```python
from build123d import *

# Parameters (mm, degrees)
SKIZZE2_W                       = 315
SKIZZE2_H                       = 50
AUFSATZ_LINEAR_AUSTRAGEN1_DEPTH = 85
SKIZZE4_W                       = 295
SKIZZE4_H                       = 55
SCHNITT_LINEAR_AUSTRAGEN1_DEPTH = 30
VERRUNDUNG1_R                   = 10
VERRUNDUNG2_R                   = 10
VERRUNDUNG3_R                   = 10
VERRUNDUNG4_R                   = 10
SKIZZE11_W                      = 45
SKIZZE11_H                      = 5
SKIZZE11_H_2                    = 5.008661904
SCHNITT_LINEAR_AUSTRAGEN4_DEPTH = 1.6
SKIZZE13_W                      = 295
SKIZZE13_H                      = 3
AUFSATZ_LINEAR_AUSTRAGEN2_DEPTH = 4.2
SKIZZE14_W                      = 8
SKIZZE14_H                      = 4
SCHNITT_LINEAR_AUSTRAGEN5_DEPTH = 19
SKIZZE15_W                      = 50
SKIZZE15_H                      = 1.5
AUFSATZ_LINEAR_AUSTRAGEN3_DEPTH = 2
SKIZZE16_W                      = 50
SKIZZE16_H                      = 1.5
AUFSATZ_LINEAR_AUSTRAGEN4_DEPTH = 2
SKIZZE17_R                      = 2.3
SCHNITT_LINEAR_AUSTRAGEN6_DEPTH = 4
SKIZZE19_W                      = 182.800022846
SKIZZE19_H                      = 85
SCHNITT_LINEAR_AUSTRAGEN8_DEPTH = 80


with BuildPart() as part:
    # Skizze2 → Aufsatz-Linear austragen1 (new body)
    with BuildSketch(Plane.XY):
        with Locations((157.5, 25)):
            Rectangle(SKIZZE2_W, SKIZZE2_H)
    extrude(amount=AUFSATZ_LINEAR_AUSTRAGEN1_DEPTH)

    # Skizze4 → Schnitt-Linear austragen1 (cut)
    with BuildSketch(Plane(origin=(0, 50, 0), x_dir=(1, 0, 0), z_dir=(0, 1, 0))):
        with Locations((157.5, -42.5)):
            Rectangle(SKIZZE4_W, SKIZZE4_H)
    extrude(amount=-SCHNITT_LINEAR_AUSTRAGEN1_DEPTH, mode=Mode.SUBTRACT)

    # Verrundung1
    verrundung1_edges = [part.edges().sort_by_distance(p)[0] for p in [
        (315, 25, 0),
    ]]
    fillet(verrundung1_edges, radius=VERRUNDUNG1_R)

    # Verrundung2
    verrundung2_edges = [part.edges().sort_by_distance(p)[0] for p in [
        (315, 25, 85),
    ]]
    fillet(verrundung2_edges, radius=VERRUNDUNG2_R)

    # Verrundung3
    verrundung3_edges = [part.edges().sort_by_distance(p)[0] for p in [
        (0, 25, 85),
    ]]
    fillet(verrundung3_edges, radius=VERRUNDUNG3_R)

    # Verrundung4
    verrundung4_edges = [part.edges().sort_by_distance(p)[0] for p in [
        (0, 25, 0),
    ]]
    fillet(verrundung4_edges, radius=VERRUNDUNG4_R)

    # Skizze11 → Schnitt-Linear austragen4 (cut)
    with BuildSketch(Plane(origin=(0, 50, 0), x_dir=(1, 0, 0), z_dir=(0, 1, 0))):
        with Locations((32.5, -12.5)):
            Rectangle(SKIZZE11_W, SKIZZE11_H)
        with Locations((32.5, -72.5)):
            Rectangle(SKIZZE11_W, SKIZZE11_H)
        with Locations((82.5, -72.5)):
            Rectangle(SKIZZE11_W, SKIZZE11_H)
        with Locations((132.5, -72.504330952)):
            Rectangle(SKIZZE11_W, SKIZZE11_H_2)
        with Locations((182.5, -72.504330952)):
            Rectangle(SKIZZE11_W, SKIZZE11_H_2)
        with Locations((232.5, -72.5)):
            Rectangle(SKIZZE11_W, SKIZZE11_H)
        with Locations((282.5, -72.5)):
            Rectangle(SKIZZE11_W, SKIZZE11_H)
        with Locations((282.5, -12.5)):
            Rectangle(SKIZZE11_W, SKIZZE11_H)
        with Locations((232.5, -12.5)):
            Rectangle(SKIZZE11_W, SKIZZE11_H)
        with Locations((182.5, -12.5)):
            Rectangle(SKIZZE11_W, SKIZZE11_H)
        with Locations((132.5, -12.5)):
            Rectangle(SKIZZE11_W, SKIZZE11_H)
        with Locations((82.5, -12.5)):
            Rectangle(SKIZZE11_W, SKIZZE11_H)
    extrude(amount=-SCHNITT_LINEAR_AUSTRAGEN4_DEPTH, mode=Mode.SUBTRACT)

    # Skizze13 → Aufsatz-Linear austragen2 (add)
    with BuildSketch(Plane(origin=(0, 20, 0), x_dir=(1, 0, 0), z_dir=(0, 1, 0))):
        with Locations((157.5, -68.5)):
            Rectangle(SKIZZE13_W, SKIZZE13_H)
    extrude(amount=AUFSATZ_LINEAR_AUSTRAGEN2_DEPTH)

    # Skizze14 → Schnitt-Linear austragen5 (cut)
    with BuildSketch(Plane.ZY.offset(-305)):
        with Locations((35, 24.4)):
            Rectangle(SKIZZE14_W, SKIZZE14_H)
    extrude(amount=-SCHNITT_LINEAR_AUSTRAGEN5_DEPTH, mode=Mode.SUBTRACT)

    # Skizze15 → Aufsatz-Linear austragen3 (add)
    with BuildSketch(Plane.XY.offset(15)):
        with Locations((280, 23.45)):
            Rectangle(SKIZZE15_W, SKIZZE15_H)
    extrude(amount=AUFSATZ_LINEAR_AUSTRAGEN3_DEPTH)

    # Skizze16 → Aufsatz-Linear austragen4 (add)
    with BuildSketch(Plane(origin=(0, 0, 67), x_dir=(-1, 0, 0), z_dir=(0, 0, -1))):
        with Locations((-280, 23.45)):
            Rectangle(SKIZZE16_W, SKIZZE16_H)
    extrude(amount=AUFSATZ_LINEAR_AUSTRAGEN4_DEPTH)

    # Skizze17 → Schnitt-Linear austragen6 (cut)
    with BuildSketch(Plane(origin=(0, 50, 0), x_dir=(1, 0, 0), z_dir=(0, 1, 0))):
        with Locations(Location((50, -80, 0), (0, 0, 270))):
            Circle(SKIZZE17_R)
        with Locations(Location((15, -80, 0), (0, 0, 270))):
            Circle(SKIZZE17_R)
        with Locations(Location((15, -5, 0), (0, 0, 270))):
            Circle(SKIZZE17_R)
        with Locations(Location((50, -5, 0), (0, 0, 270))):
            Circle(SKIZZE17_R)
        with Locations(Location((65, -5, 0), (0, 0, 270))):
            Circle(SKIZZE17_R)
        with Locations(Location((99.834927097, -5, 0), (0, 0, 270))):
            Circle(SKIZZE17_R)
        with Locations(Location((65, -80, 0), (0, 0, 270))):
            Circle(SKIZZE17_R)
        with Locations(Location((100, -80, 0), (0, 0, 270))):
            Circle(SKIZZE17_R)
        with Locations(Location((114.145512134, -79.164010762, 0), (0, 0, 270))):
            Circle(SKIZZE17_R)
        with Locations(Location((150, -80, 0), (0, 0, 270))):
            Circle(SKIZZE17_R)
        with Locations(Location((165, -80, 0), (0, 0, 270))):
            Circle(SKIZZE17_R)
        with Locations(Location((200, -80, 0), (0, 0, 270))):
            Circle(SKIZZE17_R)
        with Locations(Location((215, -80, 0), (0, 0, 270))):
            Circle(SKIZZE17_R)
        with Locations(Location((250, -80, 0), (0, 0, 270))):
            Circle(SKIZZE17_R)
        with Locations(Location((265, -80, 0), (0, 0, 270))):
            Circle(SKIZZE17_R)
        with Locations(Location((300, -80, 0), (0, 0, 270))):
            Circle(SKIZZE17_R)
        with Locations(Location((300, -5, 0), (0, 0, 270))):
            Circle(SKIZZE17_R)
        with Locations(Location((265, -5, 0), (0, 0, 270))):
            Circle(SKIZZE17_R)
        with Locations(Location((250, -5, 0), (0, 0, 270))):
            Circle(SKIZZE17_R)
        with Locations(Location((215, -5, 0), (0, 0, 270))):
            Circle(SKIZZE17_R)
        with Locations(Location((200, -5, 0), (0, 0, 270))):
            Circle(SKIZZE17_R)
        with Locations(Location((165, -5, 0), (0, 0, 270))):
            Circle(SKIZZE17_R)
        with Locations(Location((150, -5, 0), (0, 0, 270))):
            Circle(SKIZZE17_R)
        with Locations(Location((115, -5, 0), (0, 0, 270))):
            Circle(SKIZZE17_R)
    extrude(amount=-SCHNITT_LINEAR_AUSTRAGEN6_DEPTH, mode=Mode.SUBTRACT)

    # Skizze19 → Schnitt-Linear austragen8 (cut)
    with BuildSketch(Plane(origin=(0, 50, 0), x_dir=(1, 0, 0), z_dir=(0, 1, 0))):
        with Locations((248.900011423, -42.5)):
            Rectangle(SKIZZE19_W, SKIZZE19_H)
    extrude(amount=-SCHNITT_LINEAR_AUSTRAGEN8_DEPTH, mode=Mode.SUBTRACT)


solid = part.part
```
Verification items for the finished model (mm, model axes). A direction names the side the tool comes from. Coordinates: 2 decimals unless noted, no trailing zeros. Loops run counter-clockwise (first coordinate to the right, second up) from the corner with the lowest first, then second, coordinate; pieces in that order, holes last. Notation, with made-up numbers: (-22.75, 40) -> (33.25, 40) arc R5 ccw to (33.25, 44) -> close; hole circle Ø4 at (44.5, 14). An arc over 180 degrees is marked (long way). Answer in a Markdown table with one row per item. Add a question column.
1. Depth check by flat-ended pin: P1, Ø9, axis at y = 35, z = 36, coming from the +X side; P2, Ø3, axis at x = 50, z = 5, coming from the +Y side; P3, Ø5.5, axis at x = 134, z = 72, coming from the +Y side. Enter the tip coordinate at first touch or a pass-through.
2. Section check B-B, the plane y = 21.5. Enter the section's corners in (x, z).
3. Material ranges on probe 1 along Z at (x, y) = (89, 21); probe 2 along Z at (x, y) = (129.5, 46.5); probe 3 along Y at (x, z) = (25.5, 65), recorded low to high. Write a range as [from, to].
4. Section check C-C, the plane z = 73. Enter the section's corners in (x, y), then the cut area to 3 significant figures.
5. Access from +Z, -Z, +X, -X, +Y, -Y to the whole of each face (thin tool, end or side, straight path). Record for faces 4 (the face through (100, 46, 80)), 5 (the face through (3.01, 25.35, 82.15)), 6 (the face through (83, 35, 15)).
6. Section check A-A, the plane x = 131. Enter the section's corners in (y, z), then the cut area to 3 significant figures.
7. Section check D-D, the plane x = 87. Enter the section's corners in (y, z).
8. Draft check along X on faces 1 (the face through (2.85, 25.35, 3.01)), 2 (the face through (83, 25, 85)), 3 (the face through (102.115, 48.028, 4.701)). Enter one of: +X half, -X half, draft (parallel to the pull), parting line (faces both ways), or undercut.
Derived:
| question | item | result |
|---|---|---|
| 1 | P1 | stops at x = 10 |
| 1 | P2 | stops at y = 46 |
| 1 | P3 | stops at y = 48.4 |
| 2 | outline | (0, 10) arc R10 ccw to (10, 0) -> (157.5, 0) -> (157.5, 15) -> (10, 15) -> (10, 67) -> (157.5, 67) -> (157.5, 85) -> (10, 85) arc R10 ccw to (0, 75) -> close |
| 3 | probe 1 | z = [0, 15], [67, 85] |
| 3 | probe 2 | z = [0, 15], [70, 85] |
| 3 | probe 3 | y = [0, 20] |
| 4 | outline | (0, 0) -> (157.5, 0) -> (157.5, 50) -> (155, 50) -> (155, 48.4) -> (110, 48.4) -> (110, 50) -> (105, 50) -> (105, 48.4) -> (60, 48.4) -> (60, 50) -> (55, 50) -> (55, 48.4) -> (10, 48.4) -> (10, 50) -> (0, 50) -> close |
| 4 | area | 7,660 mm² |
| 5 | face 4 | +Y |
| 5 | face 5 | +Z, -X, +Y, -Y |
| 5 | face 6 | +X, +Y |
| 6 | outline | (0, 0) -> (50, 0) -> (50, 10) -> (48.4, 10) -> (48.4, 15) -> (20, 15) -> (20, 67) -> (24.2, 67) -> (24.2, 70) -> (48.4, 70) -> (48.4, 75.01) -> (50, 75.01) -> (50, 85) -> (0, 85) -> close |
| 6 | area | 2,600 mm² |
| 7 | outline | (0, 0) -> (50, 0) -> (50, 10) -> (48.4, 10) -> (48.4, 15) -> (20, 15) -> (20, 67) -> (24.2, 67) -> (24.2, 70) -> (48.4, 70) -> (48.4, 75) -> (50, 75) -> (50, 85) -> (0, 85) -> close |
| 8 | face 1 | -X half |
| 8 | face 2 | draft |
| 8 | face 3 | undercut |
